Input: part model. Units: mm. Frame: model coordinates. A direction names the side the tool comes from. Round coordinates to 2 decimals unless told otherwise and drop trailing zeros. Loops run counter-clockwise (first coordinate to the right, second up) from the corner with the lowest first, then second, coordinate; pieces in that order, holes last. Notation, with made-up numbers: M 27,65 L 78,65 A4 ccw 78,70 Z; hole C -25.5,54 d1. An arc over 180 degrees is marked long. Return JSON: item names as keys, results as strings. Group by question number.
1) Material intervals for line 1 (Y direction, x = -23, z = -10.25); line 2 (X direction, y = -32, z = -1.25); line 3 (X direction, y = 42.5, z = -4.75), sorted ascending. Write a range as from..to.
2) Access query for faces 1 (the face through (-97.457, -49.272, -4.006)), 2 (the face through (-92.8, 54.07, -6.78)), 3 (the face through (92.694, -51.539, -0.501)). Directions: +Z, -Z, +X, -X, +Y, -Y. A direction counts if a zero-diameter tool reaches every point of the face in a straight line with its end or side. Return the directions, or none.
3) Section B-B (y = -28.5). Output: boundary loops of the cut face in (x, z).
4) Contact query for flat-ended pins moving along their axis: P1, Ø1.8, axis at x = -96.5, z = -11, coming from the +Y side; P2, Ø5, axis at y = -2, z = -9.5, coming from the -X side; P3, Ø0.7, axis at x = -97, z = -11, coming from the -Y side. Output: stop coordinate, or through.
5) Section A-A (x = -39). Output: boundary loops of the cut face in (y, z).
6) Mould query, pull axis X, two halves, no side actions, for faces 4 (the face through (-94.16, -55.6, -6.26)), 5 (the face through (92.814, 51.419, -0.501)), 6 (the face through (-1, -57.798, -6)). Classes: +X half, -X half, draft (parallel to the pull), parting line (faces both ways), or undercut.
7) Section C-C (z = -9.5). Output: boundary loops of the cut face in (x, y).
from build123d import *

# Parameters (mm, degrees)
BOSS_EXTRUDE1_DEPTH = 12.7
BOSS_EXTRUDE2_DEPTH = 1.016
CUT_EXTRUDE1_REACH  = 208.793
CUT_EXTRUDE2_DEPTH  = 153.771026153


with BuildPart() as part:
    # Sketch1 → Boss-Extrude1 (new body)
    with BuildSketch(Plane.XY):
        with BuildLine():
            Line((-99.0727, 46.0375), (-99.0727, -46.0375))
            ThreePointArc((-99.0727, -46.0375), (-95.628217168, -54.353217168), (-87.3125, -57.7977))
            Line((-87.3125, -57.7977), (87.3125, -57.7977))
            ThreePointArc((87.3125, -57.7977), (95.628217168, -54.353217168), (99.0727, -46.0375))
            Line((99.0727, -46.0375), (99.0727, 46.0375))
            ThreePointArc((99.0727, 46.0375), (95.628217168, 54.353217168), (87.3125, 57.7977))
            Line((87.3125, 57.7977), (-87.3125, 57.7977))
            ThreePointArc((-87.3125, 57.7977), (-95.628217168, 54.353217168), (-99.0727, 46.0375))
        make_face()
        with BuildLine():
            Line((87.3125, 55.7657), (-87.3125, 55.7657))
            ThreePointArc((-87.3125, 55.7657), (-94.191376189, 52.916376189), (-97.0407, 46.0375))
            Line((-97.0407, 46.0375), (-97.0407, -46.0375))
            ThreePointArc((-97.0407, -46.0375), (-94.191376189, -52.916376189), (-87.3125, -55.7657))
            Line((-87.3125, -55.7657), (87.3125, -55.7657))
            ThreePointArc((87.3125, -55.7657), (94.191376189, -52.916376189), (97.0407, -46.0375))
            Line((97.0407, -46.0375), (97.0407, 46.0375))
            ThreePointArc((97.0407, 46.0375), (94.191376189, 52.916376189), (87.3125, 55.7657))
        make_face(mode=Mode.SUBTRACT)
    extrude(amount=-BOSS_EXTRUDE1_DEPTH)

    # Sketch2 → Boss-Extrude2 (add)
    with BuildSketch(Plane.XY):
        with BuildLine():
            Line((-97.0407, 46.0375), (-97.0407, -46.0375))
            ThreePointArc((-97.0407, -46.0375), (-94.191376189, -52.916376189), (-87.3125, -55.7657))
            Line((-87.3125, -55.7657), (87.3125, -55.7657))
            ThreePointArc((87.3125, -55.7657), (94.191376189, -52.916376189), (97.0407, -46.0375))
            Line((97.0407, -46.0375), (97.0407, 46.0375))
            ThreePointArc((97.0407, 46.0375), (94.191376189, 52.916376189), (87.3125, 55.7657))
            Line((87.3125, 55.7657), (-87.3125, 55.7657))
            ThreePointArc((-87.3125, 55.7657), (-94.191376189, 52.916376189), (-97.0407, 46.0375))
        make_face()
        with BuildLine():
            Line((-95.0087, 46.0375), (-95.0087, -46.0375))
            ThreePointArc((-95.0087, -46.0375), (-92.754535209, -51.479535209), (-87.3125, -53.7337))
            Line((-87.3125, -53.7337), (87.3125, -53.7337))
            ThreePointArc((87.3125, -53.7337), (92.754535209, -51.479535209), (95.0087, -46.0375))
            Line((95.0087, -46.0375), (95.0087, 46.0375))
            ThreePointArc((95.0087, 46.0375), (92.754535209, 51.479535209), (87.3125, 53.7337))
            Line((87.3125, 53.7337), (-87.3125, 53.7337))
            ThreePointArc((-87.3125, 53.7337), (-92.754535209, 51.479535209), (-95.0087, 46.0375))
        make_face(mode=Mode.SUBTRACT)
    extrude(amount=-BOSS_EXTRUDE2_DEPTH)

    # Sketch3 → Cut-Extrude1 (cut, up to next)
    with BuildSketch(Plane.ZY.offset(99.0727), mode=Mode.PRIVATE) as cut_extrude1_sk1:
        with BuildLine():
            Line((-12.7, 50.8), (-7.637414644, 50.8))
            ThreePointArc((-7.637414644, 50.8), (-4.045312196, 49.312102448), (-2.557414644, 45.72))
            Line((-2.557414644, 45.72), (-2.557414644, -45.72))
            ThreePointArc((-2.557414644, -45.72), (-4.045312196, -49.312102448), (-7.637414644, -50.8))
            Line((-7.637414644, -50.8), (-12.7, -50.8))
            Line((-12.7, -50.8), (-12.7, 50.8))
        make_face()
    cut_extrude1_tool1 = extrude(cut_extrude1_sk1.sketch, amount=-CUT_EXTRUDE1_REACH, mode=Mode.PRIVATE) & part.part
    add(cut_extrude1_tool1.solids().sort_by_distance((-99.0727, 0, -7.671479))[0], mode=Mode.SUBTRACT)

    # Sketch4 → Cut-Extrude2 (cut, through all)
    with BuildSketch(Plane(origin=(0, 57.7977, 0), x_dir=(1, 0, 0), z_dir=(0, 1, 0))):
        with BuildLine():
            Line((-69.85, 2.667), (-57.15, 2.667))
            ThreePointArc((-57.15, 2.667), (-63.5, 6.576181866), (-69.85, 2.667))
        make_face()
        with BuildLine():
            Line((69.85, 2.667), (57.15, 2.667))
            ThreePointArc((57.15, 2.667), (63.5, 6.576181866), (69.85, 2.667))
        make_face()
    extrude(amount=-CUT_EXTRUDE2_DEPTH, mode=Mode.SUBTRACT)


solid = part.part
Returned:
{
 "1": {"line 1": "y = -57.8..-55.77, 55.77..57.8", "line 2": "x = -99.07..-97.04, 97.04..99.07", "line 3": "x = 97.04..99.07"},
 "2": {"face 1": "-Z, -X", "face 2": "-Z", "face 3": "+Z, -Z"},
 "3": {"outline": "M -99.07,-2.56 L -97.04,-2.56 L -97.04,-1.02 L -95.01,-1.02 L -95.01,0 L -99.07,0 Z; M 95.01,-1.02 L 97.04,-1.02 L 97.04,-12.7 L 99.07,-12.7 L 99.07,0 L 95.01,0 Z"},
 "4": {"P1": "stops at y = 54.38", "P2": "stops at x = 97.04", "P3": "stops at y = -53.19"},
 "5": {"outline": "M -57.8,-12.7 L -55.77,-12.7 L -55.77,-1.02 L -53.73,-1.02 L -53.73,0 L -57.8,0 Z; M 53.73,-1.02 L 55.77,-1.02 L 55.77,-12.7 L 57.8,-12.7 L 57.8,0 L 53.73,0 Z"},
 "6": {"face 4": "-X half", "face 5": "undercut", "face 6": "draft"},
 "7": {"outline": "M -98.07,-50.8 A11.76 ccw -87.31,-57.8 L 87.31,-57.8 A11.76 ccw 99.07,-46.04 L 99.07,46.04 A11.76 ccw 87.31,57.8 L -87.31,57.8 A11.76 ccw -98.07,50.8 L -95.8,50.8 A9.73 cw -87.31,55.77 L 87.31,55.77 A9.73 cw 97.04,46.04 L 97.04,-46.04 A9.73 cw 87.31,-55.77 L -87.31,-55.77 A9.73 cw -95.8,-50.8 Z"}
}
